Source: CAD feature listing. Evaluate the final solid. Frame: model axes, mm. Coordinates: 2 decimals unless noted, no trailing zeros. Order: outer loops, then holes, each group sorted by start corner. A loop starts at its lowest first (then second) coordinate and runs counter-clockwise, first axis right, second up.
```python
from build123d import *

# Parameters (mm, degrees)
SKETCH1_R           = 38.1
SKETCH1_R_2         = 1.5875
SKETCH1_W           = 50.8
SKETCH1_H           = 41.91
BOSS_EXTRUDE1_DEPTH = 6.35


with BuildPart() as part:
    # Sketch1 → Boss-Extrude1 (new body)
    with BuildSketch(Plane(origin=(0, 0, 0), x_dir=(1, 0, 0), z_dir=(0, 1, 0))):
        with Locations(Location((0, 0, 0), (0, 0, 270))):
            Circle(SKETCH1_R)
        with Locations(Location((0, 33.02, 0), (0, 0, 270))):
            Circle(SKETCH1_R_2, mode=Mode.SUBTRACT)
        with Locations(Location((33.02, 0, 0), (0, 0, 270))):
            Circle(SKETCH1_R_2, mode=Mode.SUBTRACT)
        with Locations(Location((0, -33.02, 0), (0, 0, 270))):
            Circle(SKETCH1_R_2, mode=Mode.SUBTRACT)
        with Locations(Location((-33.02, 0, 0), (0, 0, 270))):
            Circle(SKETCH1_R_2, mode=Mode.SUBTRACT)
        Rectangle(SKETCH1_W, SKETCH1_H, mode=Mode.SUBTRACT)
    extrude(amount=BOSS_EXTRUDE1_DEPTH)


solid = part.part
```
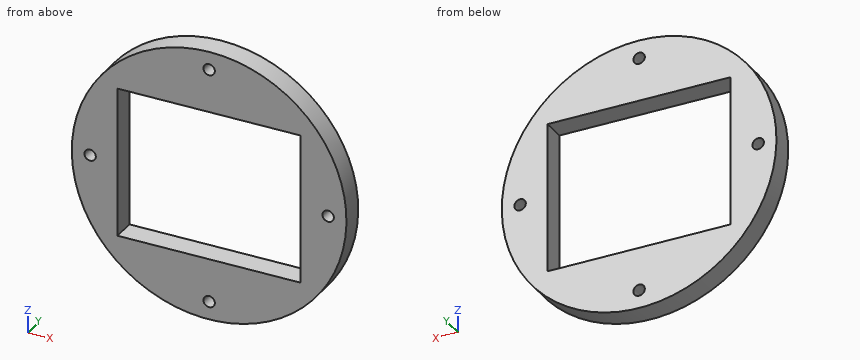
Q1. Section query C-C on z = 9. Output: boundary loops of the cut face in (x, y).
Solutions:
outline: (-37.02, 0) - (-25.4, 0) - (-25.4, 6.35) - (-37.02, 6.35) - close; (25.4, 0) - (37.02, 0) - (37.02, 6.35) - (25.4, 6.35) - close
Q2. Section query D-D on x = 0. Give the number of separate pieces and of enclosed holes in the cut face, plus the area to 3 significant figures.
Solutions:
separate pieces: 4
enclosed holes: 0
area: 177 mm2
Q3. Section query B-B on x = -21. Output: boundary loops of the cut face in (y, z) (3 decimals), plus the area to 3 significant figures.
Solutions:
outline: (0, -31.79) - (6.35, -31.79) - (6.35, -20.955) - (0, -20.955) - close; (0, 20.955) - (6.35, 20.955) - (6.35, 31.79) - (0, 31.79) - close
area: 138 mm2
Q4. Section query A-A on y = 2. Output: boundary loops of the cut face in (x, z) (1 decimal).
Solutions:
outline: circle Ø76.2 at (0, 0); hole circle Ø3.2 at (-33, 0); hole (-25.4, -21) - (25.4, -21) - (25.4, 21) - (-25.4, 21) - close; hole circle Ø3.2 at (0, -33); hole circle Ø3.2 at (0, 33); hole circle Ø3.2 at (33, 0)
Q5. Material intervals for line 1 along X through (y, z) = (5, 0); line 2 along Z through (x, y) = (0.5, 6.25) (3 decimals); line 3 along X through (y, z) = (5.5, 1), sorted ascending.
Solutions:
line 1: x = -38.1 to -34.61, -31.43 to -25.4, 25.4 to 31.43, 34.61 to 38.1
line 2: z = -38.097 to -34.527, -31.513 to -20.955, 20.955 to 31.513, 34.527 to 38.097
line 3: x = -38.09 to -34.25, -31.79 to -25.4, 25.4 to 31.79, 34.25 to 38.09
Q6. Pin query (flat end, axial travel): P1, Ø4, axis at x = 0, z = 33.02, coming from the -Y side; P2, Ø1, axis at y = 3, z = -7, coming from the -X side; P3, Ø1, axis at x = 19, y = 4.5, coming from the -Z side; P4, Ø2, axis at x = -1.5, y = 1.5, coming from the -Z side. Return the tip coordinate at first contact, or that it passes through.
Solutions:
P1: stops at y = 0
P2: stops at x = -37.54
P3: stops at z = -33.31
P4: stops at z = -38.1
